Geometry check sheet. Reference: the model listing, model coordinates, mm. A direction names the side the tool comes from. Give positions to 0.01 mm unless a question says otherwise; leave off trailing zeros. Write each loop counter-clockwise with the first axis right and the second up, starting at its lowest first coordinate (ties: lowest second). Pieces come first, ordered by that corner, then holes. Notation, with made-up numbers: M 1.25,-4.5 L 16.25,-4.5 A18 ccw 16.25,0.5 Z; hole C -36.5,63.5 d9. An arc over 180 degrees is marked long. Write each question's results on one line, items separated by ' | '.
```python
from build123d import *

# Parameters (mm, degrees)
EXTRUDE_1_DEPTH     = 50
FILLET_1_R          = 20
FILLET_2_R          = 5
SKETCH_2_R          = 1.75
CUT_EXTRUDE_1_DEPTH = 10
SKETCH_3_W          = 13.074735308
SKETCH_3_H          = 5
CUT_EXTRUDE_2_DEPTH = 10


with BuildPart() as part:
    # 草图1 → 凸台-拉伸1 (new body)
    with BuildSketch(Plane.XZ.offset(21.952986856)):
        Polygon((27.73572569, 121.735034283), (18.122569365, 118.980542412), (14.521144153, 131.549489855), (4.715724701, 128.739908146), (-21.141245178, 218.980542412), (-122.460743693, 218.980542412), (-122.460743693, 233.980542412), (122.460743693, 233.980542412), (122.460743693, 218.980542412), (-0.12837561, 218.980542412), align=None)
    extrude(amount=-EXTRUDE_1_DEPTH)

    # 圆角1
    fillet_1_edges = [part.edges().sort_by_distance(p)[0] for p in [
        (-21.141245178, 3.047013144, 218.980542412),
        (-0.12837561, 3.047013144, 218.980542412),
    ]]
    fillet(fillet_1_edges, radius=FILLET_1_R)

    # 圆角2
    fillet_2_edges = [part.edges().sort_by_distance(p)[0] for p in [
        (-122.460743693, 3.047013144, 218.980542412),
        (-122.460743693, 3.047013144, 233.980542412),
        (122.460743693, 3.047013144, 233.980542412),
        (122.460743693, 3.047013144, 218.980542412),
    ]]
    fillet(fillet_2_edges, radius=FILLET_2_R)

    # 草图2 → 切除-拉伸1 (cut)
    with BuildSketch(Plane(origin=(57.866012783, 0, 16.580554444), x_dir=(0.275449187, 0, -0.961315633), z_dir=(0.961315633, 0, 0.275449187))):
        with Locations((-117.460743693, -9)):
            Circle(SKETCH_2_R)
        with Locations((-117.460743693, 1)):
            Circle(SKETCH_2_R)
        with Locations((-117.460743693, 11)):
            Circle(SKETCH_2_R)
        with Locations((-117.460743693, 21)):
            Circle(SKETCH_2_R)
    extrude(amount=-CUT_EXTRUDE_1_DEPTH, mode=Mode.SUBTRACT)

    # 草图3 → 切除-拉伸2 (cut)
    with BuildSketch(Plane(origin=(57.866012783, 0, 16.580554444), x_dir=(0.275449187, 0, -0.961315633), z_dir=(0.961315633, 0, 0.275449187))):
        with Locations((-115.923376039, -19.452986856)):
            Rectangle(SKETCH_3_W, SKETCH_3_H)
    extrude(amount=-CUT_EXTRUDE_2_DEPTH, mode=Mode.SUBTRACT)


solid = part.part
```
Q1. Material ranges on probe 1 along Z at (x, y) = (-46.5, 2); probe 2 along X at (y, z) = (11, 143.5); probe 3 along X at (y, z) = (-3, 199), recorded low to high. Write a range as [from, to].
Answer key:
probe 1: z = [218.98, 233.98] | probe 2: x = [0.49, 21.5] | probe 3: x = [-15.42, 6.41]
Q2. Section check D-D (z = 214). Enter the section's corners in (x, y).
Answer key:
outline: M -23.01,-21.95 L 13.2,-21.95 L 13.2,28.05 L -23.01,28.05 Z
Q3. Depth check by flat-ended pin: P1, Ø15, axis at x = -60, y = -2, coming from the -Z side; P2, Ø5, axis at y = 8.5, z = 206, coming from the +X side; P3, Ø12, axis at y = 6, z = 145, coming from the -X side; P4, Ø6, axis at y = 11, z = 221.5, coming from the -X side. Enter the tip coordinate at first touch or a pass-through.
Answer key:
P1: stops at z = 218.98 | P2: stops at x = 8.82 | P3: stops at x = -1.66 | P4: stops at x = -122.46
Q4. Section check C-C (x = -84.5). Enter the section's corners in (y, z), then the cut area to 3 significant figures.
Answer key:
outline: M -21.95,218.98 L 28.05,218.98 L 28.05,233.98 L -21.95,233.98 Z | area: 750 mm2
Q5. Access from +Z, -Z, +X, -X, +Y, -Y to the whole of each face (thin tool, end or side, straight path). Record for faces 4 (the face through (21, -16.953, 127)), 5 (the face through (-121.03, 3.4, 232.48)), 6 (the face through (-76, 3, 218.981)).
Answer key:
face 4: -Z, +X, -Y | face 5: +Z, -X, +Y, -Y | face 6: -Z, -X, +Y, -Y
Q6. Section check A-A (y = -14). Enter the section's corners in (x, z), then the cut area to 3 significant figures.
Answer key:
outline: M -122.46,223.98 A5 ccw -117.46,218.98 L -36.22,218.98 A20 cw -16.99,204.49 L 4.72,128.74 L 14.52,131.55 L 18.12,118.98 L 27.74,121.74 L 7.18,193.47 A20 cw 26.41,218.98 L 117.46,218.98 A5 ccw 122.46,223.98 L 122.46,228.98 A5 ccw 117.46,233.98 L -117.46,233.98 A5 ccw -122.46,228.98 Z | area: 5,820 mm2
Q7. Section check B-B (x = 11). Enter the section's corners in (y, z), then the cut area to 3 significant figures.
Answer key:
outline: M -21.95,130.54 L 28.05,130.54 L 28.05,180.14 L -21.95,180.14 Z; M -21.95,211.73 L 28.05,211.73 L 28.05,233.98 L -21.95,233.98 Z | area: 3,590 mm2
Q8. Release check for a two-part mould opening along Z. For faces 1 (the face through (1, -21.953, 209)), 2 (the face through (16.347, 5.232, 125.177)), 3 (the face through (10.59, 3.4, 211.22)) record: released by +Z, released by -Z, zero draft, split by the parting line, or undercut.
Answer key:
face 1: zero draft | face 2: released by -Z | face 3: undercut
